from build123d import *

# Parameters (mm, degrees)
ESQUISSE1_W             = 63
ESQUISSE1_H             = 38
BOSS_EXTRU_1_DEPTH      = 900
ESQUISSE2_W             = 37
ESQUISSE2_H             = 19
ENL_V_MAT_EXTRU_1_DEPTH = 904.002214837
ESQUISSE3_R             = 5
ENL_V_MAT_EXTRU_2_DEPTH = 903.402349288


with BuildPart() as part:
    # Esquisse1 → Boss.-Extru.1 (new body)
    with BuildSketch(Plane.XY):
        with Locations((31.5, 19)):
            Rectangle(ESQUISSE1_W, ESQUISSE1_H)
    extrude(amount=BOSS_EXTRU_1_DEPTH)

    # Esquisse2 → Enlèv. mat.-Extru.1 (cut, through all)
    with BuildSketch(Plane.ZY):
        with Locations((18.5, 28.5)):
            Rectangle(ESQUISSE2_W, ESQUISSE2_H)
        with Locations((881.5, 28.5)):
            Rectangle(ESQUISSE2_W, ESQUISSE2_H)
    extrude(amount=-ENL_V_MAT_EXTRU_1_DEPTH, mode=Mode.SUBTRACT)

    # Esquisse3 → Enlèv. mat.-Extru.2 (cut, through all)
    with BuildSketch(Plane(origin=(0, 19, 0), x_dir=(1, 0, 0), z_dir=(0, 1, 0))):
        with Locations(Location((15, -18.5, 0), (0, 0, 270))):
            Circle(ESQUISSE3_R)
        with Locations(Location((48, -18.5, 0), (0, 0, 90))):
            Circle(ESQUISSE3_R)
        with Locations(Location((48, -881.5, 0), (0, 0, 270))):
            Circle(ESQUISSE3_R)
        with Locations(Location((15, -881.5, 0), (0, 0, 90))):
            Circle(ESQUISSE3_R)
    extrude(amount=-ENL_V_MAT_EXTRU_2_DEPTH, mode=Mode.SUBTRACT)


solid = part.part
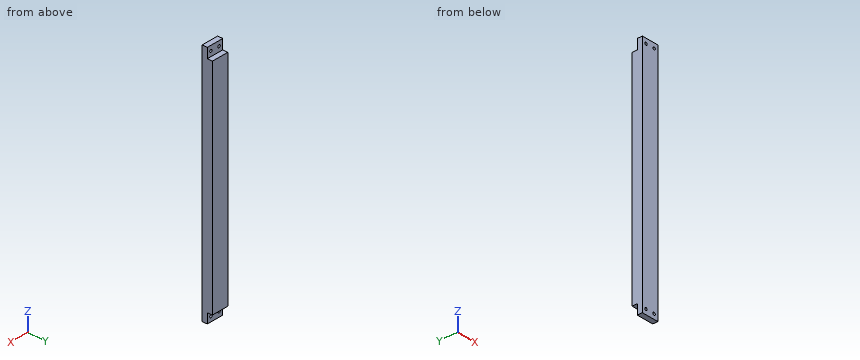
Input: part model. Units: mm. Frame: model coordinates. Coordinates: 2 decimals unless noted, no trailing zeros. Loops run counter-clockwise (first coordinate to the right, second up) from the corner with the lowest first, then second, coordinate; pieces in that order, holes last. Notation, with made-up numbers: (65, 45.25) -> (120, 45.25) arc R25 ccw to (120, 79.25) -> close; hole circle Ø9 at (29, 86). An arc over 180 degrees is marked (long way). Write item = value, one per line. Start each with the question number.
Item 1: First-contact query: P1, Ø1, axis at x = 19.5, y = 13, coming from the -Z side; P2, Ø8, axis at x = 15, z = 18.5, coming from the -Y side; P3, Ø15, axis at x = 43, y = 27, coming from the -Z side; P4, Ø13, axis at x = 15, z = 881.5, coming from the +Y side. Flat tips, straight axial feed; report the tip coordinate or a pass-through.
Item 2: Material intervals for line 1 (X direction, y = 9, z = 881); line 2 (Z direction, x = 46, y = 17.5); line 3 (Z direction, x = 46, y = 32.5), sorted ascending.
Item 3: Cut plane A-A, the plane x = 34. Return loops of the section in (y, z).
Item 4: Cut plane B-B, the plane y = 26. Return loops of the section in (x, z).
Ans:
q1.P1 = 0
q1.P2 = through
q1.P3 = 37
q1.P4 = 19
q2.line_1 = 0 to 10.03, 19.97 to 43.03, 52.97 to 63
q2.line_2 = 0 to 13.92, 23.08 to 876.92, 886.08 to 900
q2.line_3 = 37 to 863
q3.outline = (0, 0) -> (19, 0) -> (19, 37) -> (38, 37) -> (38, 863) -> (19, 863) -> (19, 900) -> (0, 900) -> close
q4.outline = (0, 37) -> (63, 37) -> (63, 863) -> (0, 863) -> close
